```python
from build123d import *

# Parameters (mm, degrees)
F0_W      = 304.8
F0_H      = 69.85
F1_DEPTH  = 38.1
F3_DEPTH  = 50.8
F4_R      = 9.525
F5_DEPTH  = 54.102
F7_DEPTH  = 127
F10_DEPTH = 76.2
F11_R     = 0.8255
F12_DEPTH = 76.2
F13_R     = 0.8303429156
F14_DEPTH = 76.2


with BuildPart() as f1:
    # F0 (on Front) → F1 (new body)
    with BuildSketch(Plane.XZ):
        with Locations((47.9073338211, -25.1322889625)):
            Rectangle(F0_W, F0_H)
    extrude(amount=-F1_DEPTH)

    # F2 (on face) → F3 (cut)
    with BuildSketch(Plane.XZ):
        Polygon((200.3073338211, 9.7927110375), (-104.4926661789, 9.7927110375), (200.3073338211, -44.1822889625), align=None)
    extrude(amount=-F3_DEPTH, mode=Mode.SUBTRACT)

    # F4 (on face) → F5 (cut)
    with BuildSketch(Plane(origin=(-104.4926661789, 0, 0), x_dir=(0, -1, 0), z_dir=(-1, 0, 0))):
        with Locations((-19.05, -25.1322889625)):
            Circle(F4_R)
    extrude(amount=-F5_DEPTH, mode=Mode.SUBTRACT)

    # F6 (on face) → F7 (cut)
    with BuildSketch(Plane(origin=(-1.4957050092, 0, -8.4463341696), x_dir=(0.9846801257, 0, -0.1743704389), z_dir=(0.1743704389, 0, 0.9846801257))):
        Polygon((161.8607493793, 38.1), (0, 38.1), (23.7803746896, 29.1751033832), (138.0803746896, 29.1751033832), align=None)
        Polygon((23.7803746896, 8.9248966168), (0, 0), (161.8607493793, 0), (138.0803746896, 8.9248966168), align=None)
    extrude(amount=-F7_DEPTH, mode=Mode.SUBTRACT)

    # F8 (on face) + F9 (on Front) → F10 (cut)
    with BuildSketch(Plane.XZ):
        with BuildLine():
            Line((-104.4926661789, 9.7927110375), (-104.4926661789, -7.0267124102))
            add(Edge.make_bspline(
                [(-104.4926661789, -7.0267124102), (-86.5421169112, -5.598796544), (-51.2128417473, -2.7884517576), (-19.0416161066, -13.0937231046), (-3.2163576046, -18.1629605909)],
                knots=[0, 0, 0, 0, 0.5080927696, 1, 1, 1, 1], degree=3))
            Line((-3.2163576046, -18.1629605909), (-1.4957050092, -8.4463341696))
            Line((-1.4957050092, -8.4463341696), (-104.4926661789, 9.7927110375))
        make_face()
    with BuildSketch(Plane.XZ):
        with BuildLine():
            ThreePointArc((-3.2163576046, -18.1629605909), (8.2323547856, -21.6399019905), (19.734878598, -24.9344555011))
            Line((19.734878598, -24.9344555011), (21.9203573303, -12.5929285423))
            Line((21.9203573303, -12.5929285423), (-1.4957050092, -8.4463341696))
            Line((-1.4957050092, -8.4463341696), (-3.2163576046, -18.1629605909))
        make_face()
        with BuildLine():
            Line((157.8853580419, -36.6700640849), (155.6058786995, -49.5424180184))
            ThreePointArc((155.6058786995, -49.5424180184), (177.93744088, -51.1635043768), (200.3073338211, -52.1197889625))
            Line((200.3073338211, -52.1197889625), (200.3073338211, -44.1822889625))
            Line((200.3073338211, -44.1822889625), (157.8853580419, -36.6700640849))
        make_face()
        with BuildLine():
            Line((134.4692957023, -32.5234697123), (131.8903467665, -47.086946056))
            ThreePointArc((131.8903467665, -47.086946056), (143.7383916941, -48.4085701416), (155.6058786995, -49.5424180184))
            Line((155.6058786995, -49.5424180184), (157.8853580419, -36.6700640849))
            Line((157.8853580419, -36.6700640849), (134.4692957023, -32.5234697123))
        make_face()
        with BuildLine():
            Line((21.9203573303, -12.5929285423), (19.734878598, -24.9344555011))
            ThreePointArc((19.734878598, -24.9344555011), (75.3915150532, -38.1426688122), (131.8903467665, -47.086946056))
            Line((131.8903467665, -47.086946056), (134.4692957023, -32.5234697123))
            Line((134.4692957023, -32.5234697123), (21.9203573303, -12.5929285423))
        make_face()
    extrude(amount=-F10_DEPTH, mode=Mode.SUBTRACT)

    # F11 (on Front) → F12 (cut)
    with BuildSketch(Plane.XZ):
        with Locations((142.7114277425, -54.1861406792)):
            Circle(F11_R)
    extrude(amount=-F12_DEPTH, mode=Mode.SUBTRACT)

    # F13 (on Front) → F14 (cut)
    with BuildSketch(Plane.XZ):
        with Locations((-34.0031449204, -53.7072889625)):
            Circle(F13_R)
    extrude(amount=-F14_DEPTH, mode=Mode.SUBTRACT)


solid = f1.part
```
Model file for the job. Use its own axes, mm. A direction names the side the tool comes from. Coordinates: 2 decimals unless noted, no trailing zeros. Loops run counter-clockwise (first coordinate to the right, second up) from the corner with the lowest first, then second, coordinate; pieces in that order, holes last. Notation, with made-up numbers: (-12, 17.5) - (21, 17.5) arc R19 ccw to (21, 33.5) - close; hole circle Ø4 at (20, 15.25). An arc over 180 degrees is marked (long way). Answer as a JSON object with one key per item and string values. Group by question number.
(1) Cut at B-B (y = 19.5). State how many separate pieces and enclosed holes the cut face has, then the cut area to 3 significant figures.
(2) Flat gauge pins, fed straight in: pin 1 (1.9 mm diameter, centred on x = -34, z = -53.71, fed in from +Y); pin 2 (1 mm diameter, centred on x = -57.5, y = 10.5, fed in from +Z); pin 3 (17.5 mm diameter, centred on x = 97, z = -44, fed in from -Y); pin 4 (10 mm diameter, centred on x = 122.5, y = 9.5, fed in from +Z). Where does each tip first touch, or does it go through?
(3) Tool access for faces 4 (the face through (-50.391, 19, -25)), 5 (the face through (143.07, 4.4, -53.1)), 6 (the face through (200.307, 19, -56)), 7 (the face through (4.67, 33.7, -40.86)), 8 (the face through (142.742, 33.575, -53.039)): list every direction of +Z, -Z, +X, -X, +Y, -Y with a clear straight run to the whole face (end or side of a thin tool).
(4) Cut at C-C (x = 44.5). Give the cut face in (y, z).
(5) Cut at A-A (z = -29.5). Give the cut face in (x, y), then the cut area to 3 significant figures.
(6) Two-plate mould, pull along Z, no slides. Class faces 1 (the face through (4.998, 4.525, -40.919)), 2 (the face through (60, 29.175, -46)), 3 (the face through (-77.82, 21.11, -34.43)): released by +Z, released by -Z, zero draft, split by the parting line, or undercut.
(7) Probe line 1 along Y through (x, z) = (97.5, -45.5); line 2 along Z through (x, y) = (-65.5, 13); line 3 along Z through (x, y) = (-60.5, 20). List the from-to ranges inside material, lowest first.
Geometry says:
{
 "1": {"separate pieces": "1", "enclosed holes": "2", "area": "8,290 mm^2"},
 "2": {"pin 1": "stops at y = 38.1", "pin 2": "stops at z = -5.54", "pin 3": "stops at y = 8.92", "pin 4": "stops at z = -45.23"},
 "3": {"face 4": "-X", "face 5": "+Z, -Y", "face 6": "+Z, -Z, +X, +Y, -Y", "face 7": "-Z, +Y", "face 8": "+Z, +Y"},
 "4": {"outline": "(8.92, -60.06) - (29.18, -60.06) - (29.18, -31.36) - (8.92, -31.36) - close"},
 "5": {"outline": "(-104.49, 0) - (-5.22, 0) - (18.93, 8.92) - (36.95, 8.92) - (36.95, 29.18) - (18.93, 29.18) - (-5.22, 38.1) - (-104.49, 38.1) - (-104.49, 27.51) - (-50.39, 27.51) - (-50.39, 10.59) - (-104.49, 10.59) - close", "area": "3,940 mm^2"},
 "6": {"face 1": "released by -Z", "face 2": "zero draft", "face 3": "undercut"},
 "7": {"line 1": "y = 8.92 to 29.18", "line 2": "z = -60.06 to -32.49, -17.78 to -5.22", "line 3": "z = -60.06 to -34.61, -15.65 to -5.4"}
}
